```python
from build123d import *

# Parameters (mm, degrees)
SKETCH1_R           = 10.416666668
SKETCH1_R_2         = 10.416666667
BOSS_EXTRUDE1_DEPTH = 65
FILLET1_R           = 2
BOSS_EXTRUDE2_DEPTH = 74
BOSS_EXTRUDE3_REACH = 100.947
SKETCH3_W           = 66.5
SKETCH3_H           = 1.5
SKETCH4_R           = 1.9
BOSS_EXTRUDE4_DEPTH = 3
SKETCH5_W           = 4
SKETCH5_H           = 8
CUT_EXTRUDE1_DEPTH  = 10
BOSS_EXTRUDE5_START = -26
BOSS_EXTRUDE5_DEPTH = 22
BOSS_EXTRUDE6_DEPTH = 17.5
FILLET2_R           = 1.5
SKETCH8_W           = 5.7
SKETCH8_H           = 0.83
CUT_EXTRUDE4_DEPTH  = 9.416666667


with BuildPart() as part:
    # Sketch1 → Boss-Extrude1 (new body)
    with BuildSketch(Plane.XY):
        with Locations((10.416666667, 10.416666667)):
            Circle(SKETCH1_R)
        with BuildLine():
            ThreePointArc((20.833333333, 10.416666667), (21.626254869, 14.402952421), (23.884304362, 17.782362305))
            ThreePointArc((23.884304363, 17.782362304), (20.833333333, 16.518608725), (17.782362304, 17.782362304))
            ThreePointArc((17.782362305, 17.782362305), (20.040411798, 14.402952421), (20.833333335, 10.416666667))
        make_face()
        with BuildLine():
            ThreePointArc((17.782362304, 3.050971029), (20.833333333, 4.314724608), (23.884304363, 3.050971029))
            ThreePointArc((23.884304362, 3.050971029), (21.626254869, 6.430380913), (20.833333333, 10.416666667))
            ThreePointArc((20.833333335, 10.416666667), (20.040411798, 6.430380912), (17.782362305, 3.050971028))
        make_face()
        with Locations((31.25, 10.416666667)):
            Circle(SKETCH1_R_2)
        with BuildLine():
            ThreePointArc((44.717637696, 3.050971029), (42.459588203, 6.430380913), (41.666666666, 10.416666667))
            ThreePointArc((41.666666667, 10.416666667), (40.873745131, 6.430380913), (38.615695638, 3.050971029))
            ThreePointArc((38.615695637, 3.050971029), (41.666666667, 4.314724608), (44.717637696, 3.050971029))
        make_face()
        with BuildLine():
            ThreePointArc((38.615695638, 17.782362305), (40.873745131, 14.402952421), (41.666666667, 10.416666667))
            ThreePointArc((41.666666666, 10.416666667), (42.459588203, 14.402952421), (44.717637696, 17.782362304))
            ThreePointArc((44.717637696, 17.782362304), (41.666666667, 16.518608725), (38.615695637, 17.782362304))
        make_face()
        with Locations((52.083333333, 10.416666667)):
            Circle(SKETCH1_R_2)
    extrude(amount=BOSS_EXTRUDE1_DEPTH)

    # Fillet1
    fillet1_edges = [part.edges().sort_by_distance(p)[0] for p in [
        (31.25, -1e-09, 65),
        (31.25, 20.833333334, 0),
        (41.666666667, 16.518608725, 0),
        (62.5, 10.416666667, 0),
        (41.666666667, 4.314724608, 0),
        (31.25, -1e-09, 0),
        (20.833333333, 4.314724608, 0),
        (41.666666667, 4.314724608, 65),
        (62.5, 10.416666667, 65),
        (41.666666667, 16.518608725, 65),
        (31.25, 20.833333334, 65),
        (20.833333333, 16.518608725, 65),
        (-1e-09, 10.416666667, 65),
        (20.833333333, 4.314724608, 65),
        (-1e-09, 10.416666667, 0),
        (20.833333333, 16.518608725, 0),
    ]]
    fillet(fillet1_edges, radius=FILLET1_R)


with BuildPart() as body_2:
    # Sketch2 → Boss-Extrude2 (new body)
    with BuildSketch(Plane(origin=(0, 0, 0), x_dir=(-1, 0, 0), z_dir=(0, 0, -1))):
        with BuildLine():
            Line((-52.083333333, 0), (-10.416666667, 0))
            ThreePointArc((-10.416666667, 0), (-3.050971029, 3.050971029), (1e-09, 10.416666667))
            Line((1e-09, 10.416666667), (2.000000001, 10.416666667))
            ThreePointArc((2.000000001, 10.416666667), (-1.636757467, 1.636757467), (-10.416666667, -2))
            Line((-10.416666667, -2), (-52.083333333, -2))
            ThreePointArc((-52.083333333, -2), (-60.863242533, 1.636757467), (-64.5, 10.416666667))
            Line((-64.5, 10.416666667), (-62.5, 10.416666667))
            ThreePointArc((-62.5, 10.416666667), (-59.449028971, 3.050971029), (-52.083333333, 0))
        make_face()
    extrude(amount=-BOSS_EXTRUDE2_DEPTH)

    # Sketch3 → Boss-Extrude3 (add, up to next)
    with BuildSketch(Plane(origin=(0, 10.416666667, 0), x_dir=(1, 0, 0), z_dir=(0, 1, 0)), mode=Mode.PRIVATE) as boss_extrude3_sk1:
        with Locations((31.25, -0.75)):
            Rectangle(SKETCH3_W, SKETCH3_H)
    boss_extrude3_tool1 = extrude(boss_extrude3_sk1.sketch, amount=-BOSS_EXTRUDE3_REACH, mode=Mode.PRIVATE) - body_2.part
    # Sketch3 → Boss-Extrude3 (add, up to next)
    with BuildSketch(Plane(origin=(0, 10.416666667, 0), x_dir=(1, 0, 0), z_dir=(0, 1, 0)), mode=Mode.PRIVATE) as boss_extrude3_sk2:
        with Locations((31.25, -73.25)):
            Rectangle(SKETCH3_W, SKETCH3_H)
    boss_extrude3_tool2 = extrude(boss_extrude3_sk2.sketch, amount=-BOSS_EXTRUDE3_REACH, mode=Mode.PRIVATE) - body_2.part
    add(boss_extrude3_tool1.solids().sort_by_distance((31.25, 10.416667, 0.75))[0])
    add(boss_extrude3_tool2.solids().sort_by_distance((31.25, 10.416667, 73.25))[0])

    # Sketch4 → Boss-Extrude4 (add)
    # profile 1 of 4: a face of its own
    with BuildSketch(Plane(origin=(0, 10.416666667, 0), x_dir=(1, 0, 0), z_dir=(0, 1, 0))):
        with BuildLine():
            Line((28.492283553, 4.777716447), (22.214567107, -1.5))
            Line((22.214567107, -1.5), (40.285432893, -1.5))
            Line((40.285432893, -1.5), (34.007716446, 4.777716447))
            ThreePointArc((34.007716446, 4.777716447), (31.25, 5.92), (28.492283553, 4.777716447))
        make_face()
        with Locations(Location((31.25, 2.02, 0), (0, 0, 180))):
            Circle(SKETCH4_R, mode=Mode.SUBTRACT)
    # profile 2 of 4: a face of its own
    with BuildSketch(Plane(origin=(0, 10.416666667, 0), x_dir=(1, 0, 0), z_dir=(0, 1, 0))):
        with BuildLine():
            Line((73.027716447, -34.242283553), (62.5, -23.714567107))
            Line((62.5, -23.714567107), (62.5, -50.285432893))
            Line((62.5, -50.285432893), (73.027716447, -39.757716447))
            ThreePointArc((73.027716447, -39.757716447), (74.17, -37), (73.027716447, -34.242283553))
        make_face()
        with Locations(Location((70.27, -37, 0), (0, 0, 180))):
            Circle(SKETCH4_R, mode=Mode.SUBTRACT)
    # profile 3 of 4: a face of its own
    with BuildSketch(Plane(origin=(0, 10.416666667, 0), x_dir=(1, 0, 0), z_dir=(0, 1, 0))):
        with BuildLine():
            Line((0, -23.714567107), (0, -50.285432893))
            Line((0, -50.285432893), (-10.527716447, -39.757716447))
            ThreePointArc((-10.527716447, -39.757716447), (-11.67, -37), (-10.527716447, -34.242283553))
            Line((-10.527716447, -34.242283553), (0, -23.714567107))
        make_face()
        with Locations((-7.77, -37)):
            Circle(SKETCH4_R, mode=Mode.SUBTRACT)
    # profile 4 of 4: a face of its own
    with BuildSketch(Plane(origin=(0, 10.416666667, 0), x_dir=(1, 0, 0), z_dir=(0, 1, 0))):
        with BuildLine():
            Line((22.214567107, -72.5), (40.285432893, -72.5))
            Line((40.285432893, -72.5), (34.007716446, -78.777716447))
            ThreePointArc((34.007716446, -78.777716447), (31.25, -79.92), (28.492283553, -78.777716447))
            Line((28.492283553, -78.777716447), (22.214567107, -72.5))
        make_face()
        with Locations((31.25, -76.02)):
            Circle(SKETCH4_R, mode=Mode.SUBTRACT)
    extrude(amount=-BOSS_EXTRUDE4_DEPTH)

    # Sketch5 → Cut-Extrude1 (cut)
    with BuildSketch(Plane(origin=(0, 10.416666667, 0), x_dir=(1, 0, 0), z_dir=(0, 1, 0))):
        with Locations((62.5, -5.5)):
            Rectangle(SKETCH5_W, SKETCH5_H)
    extrude(amount=-CUT_EXTRUDE1_DEPTH, mode=Mode.SUBTRACT)

    # Sketch6 → Boss-Extrude5 (add)
    with BuildSketch(Plane.XY.offset(74).offset(BOSS_EXTRUDE5_START)):
        with BuildLine():
            Line((62.5, 10.416666667), (64.5, 10.416666667))
            Line((64.5, 10.416666667), (64.5, 12.416666667))
            Line((64.5, 12.416666667), (64.5, 17.771583853))
            ThreePointArc((64.5, 17.771583853), (62.560313045, 23.524119525), (57.533333333, 26.927577639))
            ThreePointArc((57.533333333, 26.927577639), (56.302877847, 26.230455486), (57, 25))
            ThreePointArc((57, 25), (60.968668193, 22.313059384), (62.5, 17.771583853))
            Line((62.5, 17.771583853), (62.5, 10.416666667))
        make_face()
    extrude(amount=-BOSS_EXTRUDE5_DEPTH)

    # Sketch6<3> → Boss-Extrude6 (add)
    with BuildSketch(Plane.XY.offset(74)):
        with BuildLine():
            Line((-2, 12.416666667), (-2, 10.416666667))
            Line((-2, 10.416666667), (0, 10.416666667))
            Line((0, 10.416666667), (0, 17.771583853))
            ThreePointArc((0, 17.771583853), (1.531331806, 22.313059384), (5.5, 25))
            ThreePointArc((5.5, 25), (6.197122153, 26.230455486), (4.966666666, 26.927577639))
            ThreePointArc((4.966666666, 26.927577639), (-0.060313045, 23.524119525), (-2, 17.771583853))
            Line((-2, 17.771583853), (-2, 12.416666667))
        make_face()
    boss_extrude6 = extrude(amount=-BOSS_EXTRUDE6_DEPTH)

    # Mirror1: Boss-Extrude6 across plane
    add(boss_extrude6.mirror(Plane.XY.offset(37)))

    # Fillet2
    # the kernel refuses this fillet: 1.5 mm, written as the material it adds along each edge
    with BuildSketch(Plane(origin=(64.5, 10.416666667, 48), x_dir=(1, 0, 0), z_dir=(0, 0, -1))) as fillet2_piece_1_section:
        with BuildLine():
            CenterArc((FILLET2_R, -FILLET2_R), FILLET2_R, 90, 90)
            Line((0, -FILLET2_R), (0, 0))
            Line((0, 0), (FILLET2_R, 0))
        make_face()
    fillet2_piece_1 = extrude(amount=22, mode=Mode.PRIVATE)
    fillet2_piece_1 = split(fillet2_piece_1, bisect_by=Plane(origin=(70.314772408, 10.761109215, 42.470660485), z_dir=(-0.7071067811865509, 0, -0.7071067811865442)), keep=Keep.TOP, mode=Mode.PRIVATE)
    fillet2_piece_1 = split(fillet2_piece_1, bisect_by=Plane(origin=(70.314772408, 10.761109215, 31.529339515), z_dir=(-0.7071067811865515, 0, 0.7071067811865436)), keep=Keep.TOP, mode=Mode.PRIVATE)
    add(fillet2_piece_1)

    # Sketch8 → Cut-Extrude4 (cut)
    with BuildSketch(Plane.XZ.offset(2)):
        with Locations((31.25, 0.415)):
            Rectangle(SKETCH8_W, SKETCH8_H)
        with Locations((31.25, 73.585)):
            Rectangle(SKETCH8_W, SKETCH8_H)
    extrude(amount=-CUT_EXTRUDE4_DEPTH, mode=Mode.SUBTRACT)


solid = body_2.part
```
Source: CAD feature listing. Evaluate the final solid. Frame: model axes, mm. A direction names the side the tool comes from. Give positions to 0.01 mm unless a question says otherwise; leave off trailing zeros. Loops run counter-clockwise (first coordinate to the right, second up) from the corner with the lowest first, then second, coordinate; pieces in that order, holes last. Notation, with made-up numbers: (80, 38.25) -> (138, 38.25) arc R33 ccw to (138, 74.25) -> close; hole circle Ø6 at (73.25, 56.5). An arc over 180 degrees is marked (long way). Put each result on its own line as item: value. Start each with the question number.
1) Draft query along Y for faces 1 (the face through (-5, 7.417, 37)), 2 (the face through (6.203, 26.209, 8.628)), 3 (the face through (29.438, 8.938, -1.449)). Return one class per face: released by +Y, released by -Y, zero draft, split by the parting line, or undercut.
2) Cut plane B-B (z = 37). Return loops of the section in (x, y).
3) Cut plane D-D (z = -2.02). Return loops of the section in (x, y), then the cut area to 3 significant figures.
4) Cut plane C-C (y = 23.25). Return loops of the section in (x, z), then the cut area to 3 significant figures.
5) Reachability of faces 4 (the face through (31, 3, 73.17)), 5 (the face through (62, 6, 9.5)), 6 (the face through (59.5, 3.1, 36.5)), 7 (the face through (1.49, 22.26, 65.37)), 8 (the face through (0, 20, 56.5)) from +Z, -Z, +X, -X, +Y, -Y: full face, straight path, thin tool, end or side. Return the list, or none.
6) Contact query for flat-ended pins moving along their axis: P1, Ø6, axis at y = 13.5, z = 36, coming from the -X side; P2, Ø6, axis at y = 2, z = 47.5, coming from the +X side; P3, Ø10, axis at x = 12, y = 12, coming from the +Z side; P4, Ø5.5, axis at x = 33.5, z = 75.5, coming from the -Y side. Output: stop coordinate, or through.
7) Cut plane A-A (x = 31.25). Return loops of the section in (y, z).
8) Material intervals for probe 1 along Z at (x, y) = (31.25, 8.55); probe 2 along Z at (x, y) = (54, 5); probe 3 along Y at (x, z) = (36, 16.5), sorted ascending.
Results are:
1. face 1: released by -Y
1. face 2: undercut
1. face 3: zero draft
2. outline: (-11.67, 7.42) -> (-9.67, 7.42) -> (-9.67, 10.42) -> (-11.67, 10.42) -> close; (-5.87, 7.42) -> (-1.63, 7.42) arc R12.42 ccw to (10.42, -2) -> (52.08, -2) arc R12.42 ccw to (64.13, 7.42) -> (68.37, 7.42) -> (68.37, 10.42) -> (66, 10.42) arc R1.5 cw to (64.5, 11.92) -> (64.5, 17.77) arc R9.5 ccw to (57.53, 26.93) arc R1 ccw to (57, 25) arc R7.5 cw to (62.5, 17.77) -> (62.5, 10.42) arc R10.42 cw to (52.08, 0) -> (10.42, 0) arc R10.42 cw to (0, 10.42) -> (-5.87, 10.42) -> close; (72.17, 7.42) -> (74.17, 7.42) -> (74.17, 10.42) -> (72.17, 10.42) -> close
3. outline: (25.73, 7.42) -> (29.35, 7.42) -> (29.35, 10.42) -> (25.73, 10.42) -> close; (33.15, 7.42) -> (36.77, 7.42) -> (36.77, 10.42) -> (33.15, 10.42) -> close
3. area: 21.7 mm2
4. outline: (-0.26, 0) -> (2.38, 0) -> (2.38, 17.5) -> (-0.26, 17.5) -> close; (-0.26, 56.5) -> (2.38, 56.5) -> (2.38, 74) -> (-0.26, 74) -> close; (60.12, 26) -> (62.76, 26) -> (62.76, 48) -> (60.12, 48) -> close
4. area: 150 mm2
5. face 4: +Z, -Y
5. face 5: +X, +Y, -Y
5. face 6: none
5. face 7: +Z, -Z, +X
5. face 8: +X, -X, +Y
6. P1: stops at x = 62.5
6. P2: stops at x = 63.26
6. P3: stops at z = 74
6. P4: stops at y = -2
7. outline: (-2, 0.83) -> (7.42, 0.83) -> (7.42, -0.12) -> (10.42, -0.12) -> (10.42, 1.5) -> (0, 1.5) -> (0, 72.5) -> (10.42, 72.5) -> (10.42, 74.12) -> (7.42, 74.12) -> (7.42, 73.17) -> (-2, 73.17) -> close; (7.42, -5.92) -> (10.42, -5.92) -> (10.42, -3.92) -> (7.42, -3.92) -> close; (7.42, 77.92) -> (10.42, 77.92) -> (10.42, 79.92) -> (7.42, 79.92) -> close
8. probe 1: z = -5.92 to -3.92, -0.12 to 1.5, 72.5 to 74.12, 77.92 to 79.92
8. probe 2: z = 0 to 1.5, 72.5 to 74
8. probe 3: y = -2 to 0
